Input: part model. Units: mm. Frame: model coordinates. Face numbers are marked on the shaded views. Round coordinates to 2 decimals unless told otherwise and drop trailing zeros. Order: outer loops, then holes, each group sorted by start corner. A loop starts at its lowest first (then second) coordinate and runs counter-clockwise, first axis right, second up. Notation, with made-up numbers: M 83,17.25 L 140,17.25 A15 cw 140,43.25 Z; hole C 20.25,19.25 d5. An arc over 180 degrees is marked long. One line per question, with ' | ' between items.
```python
from build123d import *

# Parameters (mm, degrees)
ESQUISSE2_R             = 1.65
ENL_V_MAT_EXTRU_1_DEPTH = 50.09500993
ESQUISSE3_R             = 3.35
ENL_V_MAT_EXTRU_2_DEPTH = 56.81800793


with BuildPart() as part:
    # Esquisse1 → Révolution1 (revolve)
    with BuildSketch(Plane.XY, mode=Mode.PRIVATE) as r_volution1_sk:
        with BuildLine():
            Line((12.5, 0), (15.4, 0))
            Line((15.4, 0), (15.4, 17.5))
            Line((15.4, 17.5), (7, 27))
            Line((7, 27), (7, 40))
            ThreePointArc((7, 40), (4.031128874, 42.92947553), (0, 44))
            Line((0, 44), (0, 24))
            Line((0, 24), (5.443157895, 24))
            Line((5.443157895, 24), (11.5, 17.15))
            Line((11.5, 17.15), (12.5, 17.15))
            Line((12.5, 17.15), (12.5, 0))
        make_face()
    revolve(r_volution1_sk.sketch.rotate(Axis((0, 0, 0), (0, 1, 0)), 90), axis=Axis((0, 0, 0), (0, 1, 0)))

    # Esquisse2 → Enlèv. mat.-Extru.1 (cut, through all)
    with BuildSketch(Plane.XY):
        with Locations(Location((0, 9, 0), (0, 0, 90))):
            Circle(ESQUISSE2_R)
    extrude(amount=-ENL_V_MAT_EXTRU_1_DEPTH, mode=Mode.SUBTRACT)

    # Esquisse3 → Enlèv. mat.-Extru.2 (cut, through all)
    with BuildSketch(Plane.XY.offset(-15.3)):
        with Locations((0, 9)):
            Circle(ESQUISSE3_R)
    extrude(amount=-ENL_V_MAT_EXTRU_2_DEPTH, mode=Mode.SUBTRACT)


solid = part.part
```
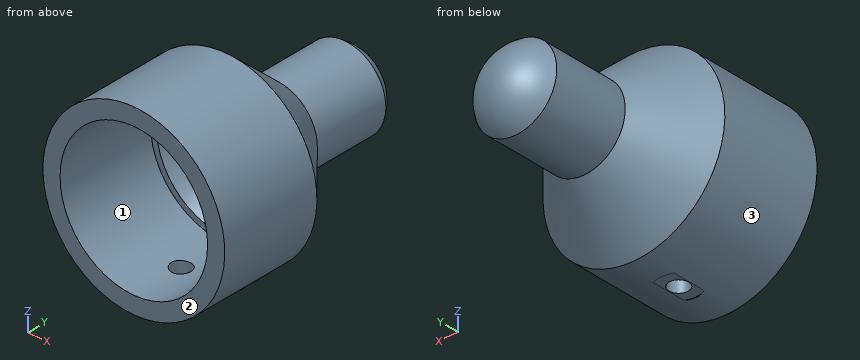
Item 1: Section query B-B, the plane z = 0. Return loops of the section in (x, y) (3 decimals), plus the area to 3 significant figures.
Report:
outline: M -15.4,0 L -12.5,0 L -12.5,17.15 L -11.5,17.15 L -5.443,24 L 5.443,24 L 11.5,17.15 L 12.5,17.15 L 12.5,0 L 15.4,0 L 15.4,17.5 L 7,27 L 7,40 A8.125 ccw -7,40 L -7,27 L -15.4,17.5 Z | area: 429 mm²
Item 2: Section query A-A, the plane x = 0. Return loops of the section in (y, z) (3 decimals), plus the area to 3 significant figures.
Report:
outline: M 0,-15.4 L 5.65,-15.4 L 5.65,-15.3 L 7.35,-15.3 L 7.35,-12.5 L 0,-12.5 Z; M 0,12.5 L 17.15,12.5 L 17.15,11.5 L 24,5.443 L 24,-5.443 L 17.15,-11.5 L 17.15,-12.5 L 10.65,-12.5 L 10.65,-15.3 L 12.35,-15.3 L 12.35,-15.4 L 17.5,-15.4 L 27,-7 L 40,-7 A8.125 ccw 40,7 L 27,7 L 17.5,15.4 L 0,15.4 Z | area: 419 mm²
Item 3: Line query: line 1 along X through (y, z) = (7, 0); line 2 along X through (y, z) = (21.5, 6); line 3 along Z through (x, y) = (-9, 6). Output: solid intervals per line, ascending. Write a range as from..to.
Report:
line 1: -15.4..-12.5, 12.5..15.4 | line 2: -10.23..-4.75, 4.75..10.23 | line 3: -12.5..-8.67, 8.67..12.5
Item 4: Section query C-C, the plane y = 16. Return loops of the section in (x, z), plus the area to 3 significant figures.
Report:
outline: C 0,0 d30.8; hole C 0,0 d25 | area: 254 mm²
Item 5: Mould query, pull axis X, two halves, no side actions, for the marked faces 1, 2 and 3. Classes: +X half, -X half, draft (parallel to the pull), parting line (faces both ways), or undercut.
Report:
face 1: undercut | face 2: draft | face 3: parting line
Item 6: First-contact query: pin 1 (5 mm diameter, centred on x = 5, y = 37.5, fed in from -Z); pin 2 (1.8 mm diameter, centred on x = -1, y = 10.5, fed in from -Z); pin 3 (4 mm diameter, centred on x = 11.5, z = -9, fed in from +Y); pin 4 (12 mm diameter, centred on x = -3.5, y = 10.5, fed in from -Z). Flat tips, straight axial feed; report the tip coordinate or a pass-through.
Report:
pin 1: z = -6.54 | pin 2: z = -15.3 | pin 3: y = 20.66 | pin 4: z = -15.4
Item 7: Section query D-D, the plane y = 9. Return loops of the section in (x, z).
Report:
outline: M -1.75,-15.3 L -1.65,-15.3 L -1.65,-12.39 A12.5 cw long 1.65,-12.39 L 1.65,-15.3 L 1.75,-15.3 A15.4 ccw long Z
